Autodesk Inventor part; units mm, degrees
ref_plane "Płaszczyzna konstrukcyjna1" through (0, 0, -11.65) normal (0, 0, 1) x (1, 0, 0)
ref_plane "YZ Plane" through (0, 0, 0) normal (1, 0, 0) x (0, 1, 0)
ref_plane "XZ Plane" through (0, 0, 0) normal (0, 1, 0) x (-1, 0, 0)
sketch "Szkic1" plane through (0, 0, 0) normal (0, 1, 0) x (-1, 0, 0)
  circle A0 centre (0, 0) radius 11.65
  dimension "d0" = 23.3
extrude "Wyciągnięcie proste1" add sketch "Szkic1" along normal blind 40
sketch "Szkic2" plane through (0, 40, 0) normal (0, 1, 0) x (1, 0, 0)
  circle A0 centre (0, 0) radius 11.65
  line L0 (0, -11.65) -> (-10, -11.65)
  arc A1 (-7.185, -9.1705) -> (0, -11.65) centre (0, 0) ccw
  line L1 (0, -11.65) -> (-7.185, -11.65)
  line L2 (0, -9.1705) -> (-7.185, -9.1705)
  line L3 (0, -11.65) -> (0, -5.8216)
  line L4 (-10, -11.65) -> (-7.185, -9.1705)
  line L5 (0, -11.65) -> (10, -11.65)
  line L6 (0, -9.1705) -> (7.185, -9.1705)
  line L7 (10, -11.65) -> (7.185, -9.1705)
  dimension "d3" = 10
  dimension "d6" = 7.185
extrude "Wyciągnięcie proste2" add sketch "Szkic2" against normal blind 30 contours A0 L0 L4 | L7 L5 A0
ref_plane "Płaszczyzna konstrukcyjna1" through (0, 0, -11.65) normal (0, 0, 1) x (1, 0, 0)
sketch "Szkic3" plane through (0, 0, -11.65) normal (0, 0, 1) x (1, 0, 0)
  circle A0 centre (8.025, 5.275) radius 3.625
  line L0 (11.65, 0) -> (-11.65, 0)
  line L1 (11.65, 8.9) -> (-11.65, 8.9)
  circle A1 centre (8.025, 5.275) radius 2
  point P0 (0, 0)
  dimension "d10" = 8.9
  dimension "d11" = 4
extrude "Wyciągnięcie proste3" add sketch "Szkic3" along normal blind 12 and the other way blind 7 contours A0 | A1
properties part number "Pomp]"
Read the model definition and answer for the solid it produces. Units are mm, in the model's axes. A direction names the side the tool comes from. Give positions to 0.01 mm unless a question says otherwise; leave off trailing zeros. Write each loop counter-clockwise with the first axis right and the second up, starting at its lowest first coordinate (ties: lowest second). Pieces come first, ordered by that corner, then holes. Notation, with made-up numbers: (-38.5, -36) - (-15.5, -36) arc R16 cw to (-15.5, -5) - close; hole circle Ø2 at (88.5, 4). An arc over 180 degrees is marked (long way). Use CSV: the item, a comma, the result in double quotes. Start each with the question number.
(1) Consider line 1 along Z through (x, y) = (-9.75, 32.5); line 2 along Z through (x, y) = (-9.25, 26); line 3 along Z through (x, y) = (1.25, 37). Determine where each line is inside the solid, lowest interval first.
(2) Given P1, Ø6, axis at y = 10.5, z = -4, coming from the -X side; P2, Ø4, axis at y = 29.5, z = -11, coming from the -X side; P3, Ø1.2, axis at x = 7.5, z = 10.5, coming from the -Y side, each flat-ended and moving along its own axis, determine where each tip first touches the part or whether it passes through.
(3) Find section D-D (x = 6). Give the vertices of the cut face in (y, z).
(4) Determine the mould class of faces 5 (the flat face through (-7, 10, 11)), 6 (the flat face through (-8.612, 25.21, 10.428)), 7 (the flat face through (0, 25, 11.65)), 8 (the flat face through (8, 5, -18.65)) for opening direction Z: +Z half, -Z half, draft (parallel to the pull), parting line (faces both ways), or undercut.
(5) For faces 1 (the cylindrical face through (11.374, 3.887, -13.339)), 2 (the flat face through (8.612, 25.21, 10.428)), 3 (the flat face through (0, 40, 0)), 4 (the flat face through (6, 10, 11)), determine the directions among +Z, -Z, +X, -X, +Y, -Y from which every point of the face is accessible in a straight line to the end or side of a thin tool.
(6) Find section A-A (x = -5.25). Give the vertices of the cut face in (y, z).
(7) Find section C-C (z = -8.5). Give the vertices of the cut face in (x, y) (3 decimals), plus the area to 3 significant figures.
Findings below:
1,line 1,"-6.38 to 6.38, 11.43 to 11.65"
1,line 2,"-7.08 to 7.08, 10.99 to 11.65"
1,line 3,"-11.58 to 11.65"
2,P1,"x = -11.61"
2,P2,"x = -7.4"
2,P3,"y = 10"
3,outline,"(0, -9.99) - (2.27, -9.99) - (2.27, -18.65) - (8.28, -18.65) - (8.28, -9.99) - (40, -9.99) - (40, 11.65) - (10, 11.65) - (10, 9.99) - (0, 9.99) - close"
4,face 5,"draft"
4,face 6,"undercut"
4,face 7,"+Z half"
4,face 8,"-Z half"
5,face 1,"-Z"
5,face 2,"+X, +Y, -Y"
5,face 3,"+Z, -Z, +X, -X, +Y"
5,face 4,"+Z, +X, -Y"
6,outline,"(0, -10.4) - (40, -10.4) - (40, 11.65) - (10, 11.65) - (10, 10.4) - (0, 10.4) - close"
7,outline,"(-7.967, 0) - (7.967, 0) - (7.967, 1.65) arc R3.625 ccw (long way) to (7.967, 8.9) - (7.967, 40) - (-7.967, 40) - close"
7,area,"658 mm2"
